For this review, take the finished solid that the model builds, in its own axes (mm). Face numbers are marked on the shaded views. A direction names the side the tool comes from. Round coordinates to 2 decimals unless told otherwise and drop trailing zeros. Loops run counter-clockwise (first coordinate to the right, second up) from the corner with the lowest first, then second, coordinate; pieces in that order, holes last.
1. Consider section D-D on y = 18. State the section outline as (x, z) points.
2. Consider section B-B on z = 97. State the section outline as (x, y) points, then the cut area to 3 significant figures.
3. Tool access review of the marked faces 1 and 2: name each direction out of +Z, -Z, +X, -X, +Y, -Y from which nothing blocks a thin tool from reaching the whole face with its end or side.
4. Clearance check with flat-ended pins moving along their axes: pin 1 Ø1 at (x, z) = (-6, 95) entering from -Y; pin 2 Ø3 at (x, y) = (-11.5, -12.5) entering from +Z; pin 3 Ø6 at (x, z) = (-14.5, 94.5) entering from -Y. State where each tip first meets the part, or that it passes through.
5. Consider section A-A on y = 57. State the section outline as (x, z) points, then the cut area to 3 significant figures.
6. Consider section C-C on y = -12.5. State the section outline as (x, z) points.
7. To check wall thickness, follow line 1 along X through (y, z) = (59, 10.5); line 2 along Z through (x, y) = (-9, 38); line 3 along Y through (x, z) = (-0.5, 113.5). State the ranges of each line that lie inside material, in increasing order.
Solid Edge part; units mm, degrees
sketch "Sketch1" plane through (0, 0, 0) normal (0, 0, 1) x (1, 0, 0)
  line L0 (-12.0351, -58.1811) -> (-23.1158, 54.7315)
  line L1 (23.1158, 54.7315) -> (12.0351, -58.1811)
  arc A0 (12.0351, -58.1811) -> (-12.0351, -58.1811) centre (0, -57) cw
  arc A1 (-23.1158, 54.7315) -> (23.1158, 54.7315) centre (0, 57) cw
extrude "Protrusion1" add sketch "Sketch1" along normal blind 13
sketch "Sketch2" plane through (0, 5.5669, 13) normal (0, 0, 1) x (0.0977, 0.9952, 0)
  circle A0 centre (51.1872, 5.0232) radius 16.0822
extrude "ExtrudedProtrusion_3" add sketch "Sketch2" along normal blind 120
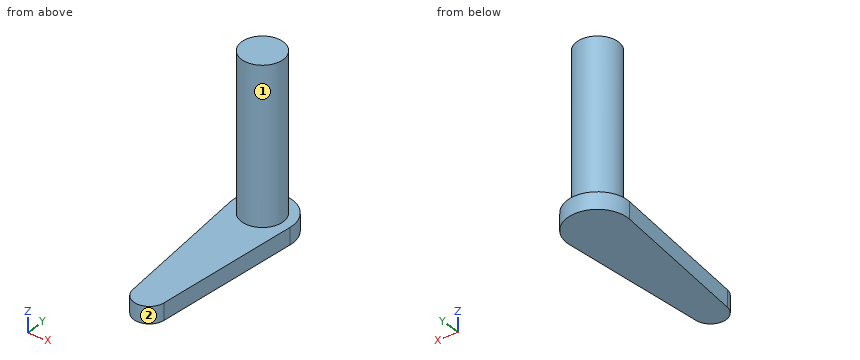
Resolved:
1. outline: (-19.51, 0) - (19.51, 0) - (19.51, 13) - (-19.51, 13) - close
2. outline: circle Ø32.16 at (0, 57)
2. area: 813 mm2
3. face 1: +Z
3. face 2: +Z, -Z, -Y
4. pin 1: stops at y = 41.89
4. pin 2: stops at z = 13
4. pin 3: stops at y = 45.76
5. outline: (-23.23, 0) - (23.23, 0) - (23.23, 13) - (16.08, 13) - (16.08, 133) - (-16.08, 133) - (-16.08, 13) - (-23.23, 13) - close
5. area: 4,460 mm2
6. outline: (-16.52, 0) - (16.52, 0) - (16.52, 13) - (-16.52, 13) - close
7. line 1: x = -23.14 to 23.14
7. line 2: z = 0 to 13
7. line 3: y = 40.93 to 73.07
